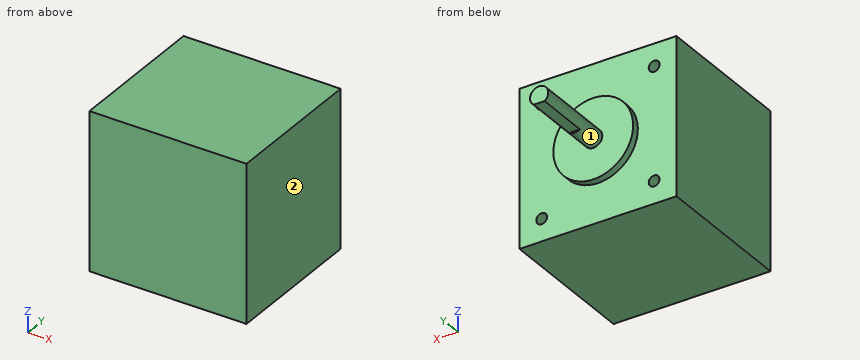
```python
from build123d import *

# Parameters (mm, degrees)
SKETCH1_W               = 43.3
SKETCH1_H               = 43.3
BOSS_EXTRUDE1_DEPTH     = 40
SKETCH2_R               = 11
BOSS_EXTRUDE2_DEPTH     = 2
SKETCH3_R               = 2.5
BOSS_EXTRUDE3_DEPTH     = 25
CUT_EXTRUDE1_DEPTH      = 72.850156576
CUT_EXTRUDE1_DEPTH_BACK = 72.850156576
SKETCH4_W               = 0.5
SKETCH4_H               = 15
SKETCH5_R               = 1.5
CUT_EXTRUDE2_DEPTH      = 4.5


with BuildPart() as part:
    # Sketch1 → Boss-Extrude1 (new body)
    with BuildSketch(Plane(origin=(0, 0, 0), x_dir=(1, 0, 0), z_dir=(0, 1, 0))):
        Rectangle(SKETCH1_W, SKETCH1_H)
    extrude(amount=BOSS_EXTRUDE1_DEPTH)

    # Sketch2 → Boss-Extrude2 (add)
    with BuildSketch(Plane(origin=(0, 40, 0), x_dir=(1, 0, 0), z_dir=(0, 1, 0))):
        with Locations(Location((0, 0, 0), (0, 0, 270))):
            Circle(SKETCH2_R)
    extrude(amount=BOSS_EXTRUDE2_DEPTH)

    # Sketch3 → Boss-Extrude3 (add)
    with BuildSketch(Plane(origin=(0, 40, 0), x_dir=(1, 0, 0), z_dir=(0, 1, 0))):
        with Locations(Location((0, 0, 0), (0, 0, 270))):
            Circle(SKETCH3_R)
    extrude(amount=BOSS_EXTRUDE3_DEPTH)

    # Sketch4 → Cut-Extrude1 (cut, two sides: drawn at the far end of the back side and taken through both)
    with BuildSketch(Plane(origin=(0, 0, 0), x_dir=(0, 0, -1), z_dir=(1, 0, 0)).offset(-CUT_EXTRUDE1_DEPTH_BACK)):
        with Locations((2.25, 57.5)):
            Rectangle(SKETCH4_W, SKETCH4_H)
    extrude(amount=CUT_EXTRUDE1_DEPTH + CUT_EXTRUDE1_DEPTH_BACK, mode=Mode.SUBTRACT)

    # Sketch5 → Cut-Extrude2 (cut)
    with BuildSketch(Plane(origin=(0, 40, 0), x_dir=(1, 0, 0), z_dir=(0, 1, 0))):
        with Locations(Location((15.5, 15.5, 0), (0, 0, 270))):
            Circle(SKETCH5_R)
        with Locations(Location((15.5, -15.5, 0), (0, 0, 270))):
            Circle(SKETCH5_R)
        with Locations(Location((-15.5, -15.5, 0), (0, 0, 270))):
            Circle(SKETCH5_R)
        with Locations(Location((-15.5, 15.5, 0), (0, 0, 270))):
            Circle(SKETCH5_R)
    extrude(amount=-CUT_EXTRUDE2_DEPTH, mode=Mode.SUBTRACT)


solid = part.part
```
Here's how the part is built. I have some questions about the finished solid (model axes, mm). Face numbers are marked on the shaded views. A direction names the side the tool comes from. Round coordinates to 2 decimals unless told otherwise and drop trailing zeros. Write each loop counter-clockwise with the first axis right and the second up, starting at its lowest first coordinate (ties: lowest second). Pieces come first, ordered by that corner, then holes.
Q1. Please list where these lines run through material, in increasing order: probe 1 along X at (y, z) = (38.2, -15.5); probe 2 along Z at (x, y) = (15, 36); probe 3 along Y at (x, z) = (-10, 13).
Q2. If we section it at C-C on y = 55: Write out the boundary of the cut face in (x, z).
Q3. If we section it at A-A on z = -15.5: Write out the boundary of the cut face in (x, y).
Q4. Will these pins go through, and if not, where does the flat tip stop? P1, Ø1.5, axis at x = -15, z = 15.5, coming from the +Y side; P2, Ø5, axis at x = 15.5, z = -15.5, coming from the +Y side; P3, Ø3.5, axis at x = 0.5, y = 57, coming from the -Z side.
Q5. If we section it at B-B on x = -15.5: Write out the boundary of the cut face in (y, z).
Q6. Which directions (+Z, -Z, +X, -X, +Y, -Y) give clear straight access to the entire face, cutting with the end or side of a thin tool? Please do the marked faces 1 and 2.
Q7. If we section it at D-D on x = -9: Write out the boundary of the cut face in (y, z).
Answer below:
1. probe 1: x = -21.65 to -17, -14 to 14, 17 to 21.65
1. probe 2: z = -21.65 to -16.91, -14.09 to 14.09, 16.91 to 21.65
1. probe 3: y = 0 to 40
2. outline: (-1.5, -2) - (1.5, -2) arc R2.5 ccw (long way) to start
3. outline: (-21.65, 0) - (21.65, 0) - (21.65, 40) - (17, 40) - (17, 35.5) - (14, 35.5) - (14, 40) - (-14, 40) - (-14, 35.5) - (-17, 35.5) - (-17, 40) - (-21.65, 40) - close
4. P1: stops at y = 35.5
4. P2: stops at y = 40
4. P3: stops at z = -2
5. outline: (0, -21.65) - (40, -21.65) - (40, -17) - (35.5, -17) - (35.5, -14) - (40, -14) - (40, 14) - (35.5, 14) - (35.5, 17) - (40, 17) - (40, 21.65) - (0, 21.65) - close
6. face 1: +Y
6. face 2: +Z, -Z, +X, +Y, -Y
7. outline: (0, -21.65) - (40, -21.65) - (40, -6.32) - (42, -6.32) - (42, 6.32) - (40, 6.32) - (40, 21.65) - (0, 21.65) - close
